The figure shows three views and two pictorial views of one solid part (mm, origin at its lowest corner). Answer the questions. Give positions to 0.01 mm unless a question says otherwise; leave off trailing zeros. Order: outer loops, then holes, each group sorted by start corner. A loop starts at its lowest first (then second) coordinate and runs counter-clockwise, first axis right, second up. Notation, with made-up numbers: (32.5, 74) - (37.5, 74) arc R24 cw to (37.5, 112) - close; hole circle Ø10 at (19.25, 5). An arc over 180 degrees is marked (long way). Answer as CSV lines item,"result". Start each with the question number.
1. Determine the mould class of the marked faces 1, 2 and 3 for opening direction Y: +Y half, -Y half, draft (parallel to the pull), parting line (faces both ways), or undercut.
2. Consider line 1 along Y through (x, z) = (50, 2.5); line 2 along Y through (x, z) = (54.05, 2) (1 decimal); line 3 along Y through (x, z) = (46.5, 3.5) (1 decimal). Determine where each line is inside the solid, lowest interval first. Write a range as [from, to].
3. Section C-C on y = 18.5 is taken. Give the vertices of the cut face in (x, z) (1 decimal).
4. Section A-A on x = 50 is taken. Give the vertices of the cut face in (y, z), and give its area (3 significant figures).
5. Section B-B on y = 50 is taken. Give the vertices of the cut face in (x, z).
6. Flat-ended cylindrical pins translate along their axes: pin 1 (1.5 mm diameter, centred on x = 86, z = 3, fed in from -Y); pin 2 (2 mm diameter, centred on y = 40.5, z = 1.5, fed in from +X); pin 3 (2 mm diameter, centred on y = 61.5, z = 3.5, fed in from +X) (1 decimal). Find the tip coordinate at first contact, or state that the pin passes through.
7. Section D-D on y = 92 is taken. Give the vertices of the cut face in (x, z), and give its area (3 significant figures).
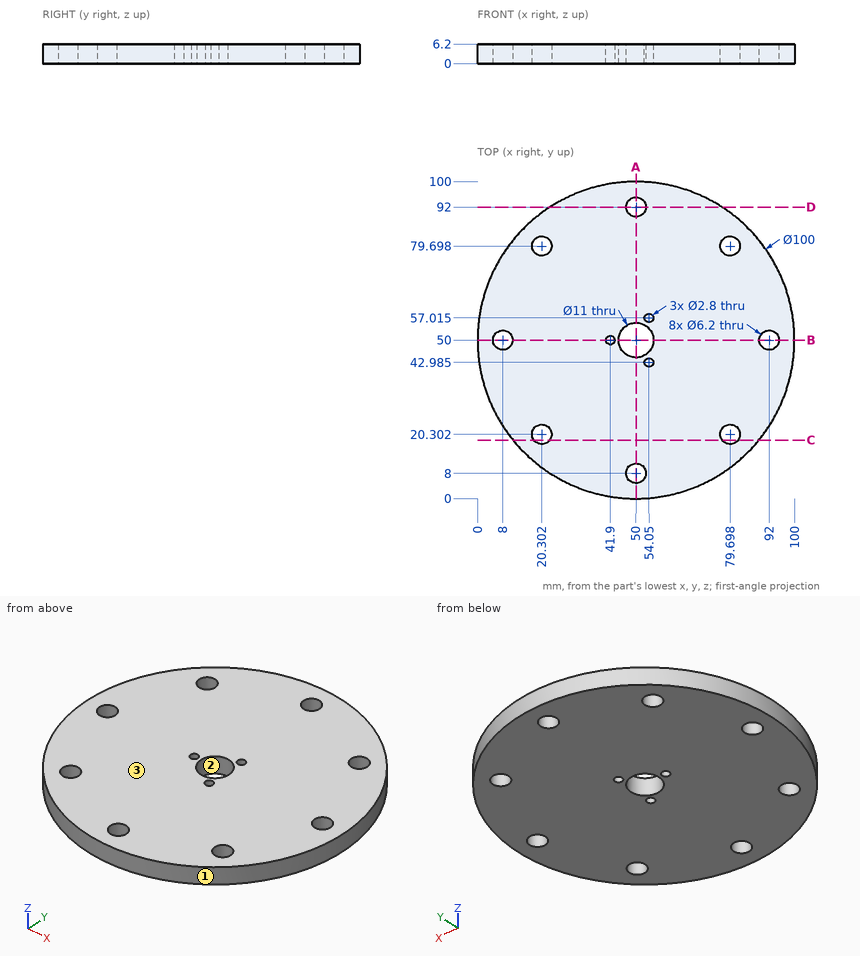
Checks:
1,face 1,"parting line"
1,face 2,"undercut"
1,face 3,"draft"
2,line 1,"y = [0, 4.9], [11.1, 44.5], [55.5, 88.9], [95.1, 100]"
2,line 2,"y = [0.2, 41.6], [44.4, 46.3], [53.7, 55.6], [58.4, 99.8]"
2,line 3,"y = [0.1, 45.8], [54.2, 99.9]"
3,outline,"(11.2, 0) - (17.8, 0) - (17.8, 6.2) - (11.2, 6.2) - close; (22.8, 0) - (77.2, 0) - (77.2, 6.2) - (22.8, 6.2) - close; (82.2, 0) - (88.8, 0) - (88.8, 6.2) - (82.2, 6.2) - close"
4,outline,"(0, 0) - (4.9, 0) - (4.9, 6.2) - (0, 6.2) - close; (11.1, 0) - (44.5, 0) - (44.5, 6.2) - (11.1, 6.2) - close; (55.5, 0) - (88.9, 0) - (88.9, 6.2) - (55.5, 6.2) - close; (95.1, 0) - (100, 0) - (100, 6.2) - (95.1, 6.2) - close"
4,area,"475 mm²"
5,outline,"(0, 0) - (4.9, 0) - (4.9, 6.2) - (0, 6.2) - close; (11.1, 0) - (40.5, 0) - (40.5, 6.2) - (11.1, 6.2) - close; (43.3, 0) - (44.5, 0) - (44.5, 6.2) - (43.3, 6.2) - close; (55.5, 0) - (88.9, 0) - (88.9, 6.2) - (55.5, 6.2) - close; (95.1, 0) - (100, 0) - (100, 6.2) - (95.1, 6.2) - close"
6,pin 1,"stops at y = 14.54"
6,pin 2,"stops at x = 99.27"
6,pin 3,"stops at x = 98.9"
7,outline,"(22.87, 0) - (46.9, 0) - (46.9, 6.2) - (22.87, 6.2) - close; (53.1, 0) - (77.13, 0) - (77.13, 6.2) - (53.1, 6.2) - close"
7,area,"298 mm²"
